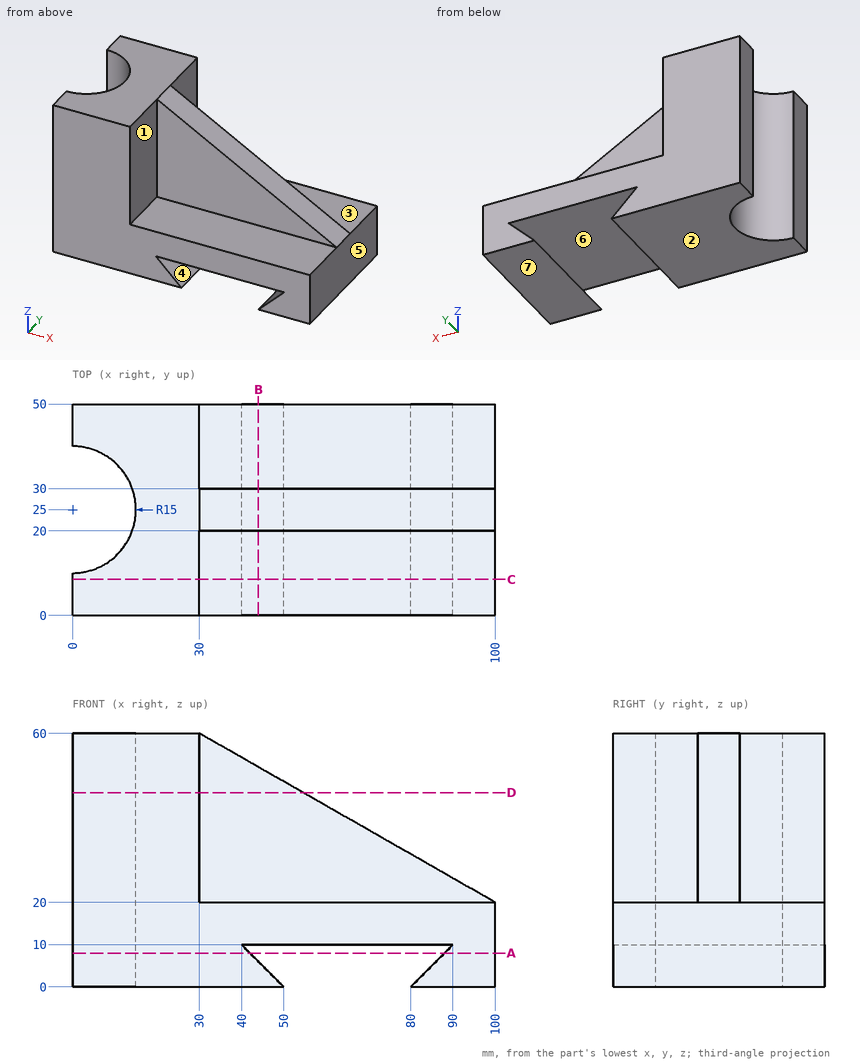
Check sheet for the drawn part. Datum: minimum x, y, z corner. Units: mm. A direction names the side the tool comes from. Coordinates: 2 decimals unless noted, no trailing zeros. Order: outer loops, then holes, each group sorted by start corner. A loop starts at its lowest first (then second) coordinate and runs counter-clockwise, first axis right, second up. Notation, with made-up numbers: (54.25, -25.5) -> (88.25, -25.5) arc R14 ccw to (88.25, -21.5) -> close; hole circle Ø5 at (14, 69.25). An arc over 180 degrees is marked (long way). Write each question's results on one line, items separated by ' | '. Start each with the question number.
1) Section check C-C (y = 8.5). Enter the section's corners in (x, z), and give its area (3 significant figures).
2) Set-up check for the marked faces 1, 2, 3 and 4: record each of +Z, -Z, +X, -X, +Y, -Y from which the full face is reachable in a straight line by a thin tool's end or side.
3) Material ranges on line 1 along Z through (x, y) = (77, 45.5); line 2 along Z through (x, y) = (40.5, 43.5); line 3 along Z through (x, y) = (47, 10), recorded low to high.
4) Section check B-B (x = 44). Enter the section's corners in (y, z).
5) Depth check by flat-ended pin: pin 1 (25 mm diameter, centred on x = 64.5, y = 33.5, fed in from -Z); pin 2 (12 mm diameter, centred on x = 62, z = 31.5, fed in from +Y); pin 3 (1.5 mm diameter, centred on y = 36.5, z = 41.5, fed in from -X). Enter the tip coordinate at first touch or a pass-through.
6) Draft check along X on the marked faces 5, 6 and 7. Enter one of: pulls with the +X half, pulls with the -X half, needs draft (parallel to the pull), parting line crosses it, or undercut.
7) Section check A-A (z = 8). Enter the section's corners in (x, y), and give its area (3 significant figures).
8) Section check D-D (z = 46). Enter the section's corners in (x, y), and give its area (3 significant figures).
Checked values:
1) outline: (0, 0) -> (50, 0) -> (40, 10) -> (90, 10) -> (80, 0) -> (100, 0) -> (100, 20) -> (30, 20) -> (30, 60) -> (0, 60) -> close | area: 2,800 mm²
2) face 1: +Z, +X, -Y | face 2: -Z, +X, -X, +Y, -Y | face 3: +Z, +X, +Y | face 4: +Y, -Y
3) line 1: 10 to 20 | line 2: 0 to 9.5, 10 to 20 | line 3: 0 to 3, 10 to 20
4) outline: (0, 0) -> (50, 0) -> (50, 6) -> (0, 6) -> close; (0, 10) -> (50, 10) -> (50, 20) -> (30, 20) -> (30, 52) -> (20, 52) -> (20, 20) -> (0, 20) -> close
5) pin 1: z = 10 | pin 2: y = 30 | pin 3: x = 8.66
6) face 5: pulls with the +X half | face 6: undercut | face 7: needs draft
7) outline: (0, 0) -> (42, 0) -> (42, 50) -> (0, 50) -> (0, 40) arc R15 cw to (0, 10) -> close; (88, 0) -> (100, 0) -> (100, 50) -> (88, 50) -> close | area: 2,350 mm²
8) outline: (0, 0) -> (30, 0) -> (30, 20) -> (54.5, 20) -> (54.5, 30) -> (30, 30) -> (30, 50) -> (0, 50) -> (0, 40) arc R15 cw to (0, 10) -> close | area: 1,390 mm²
